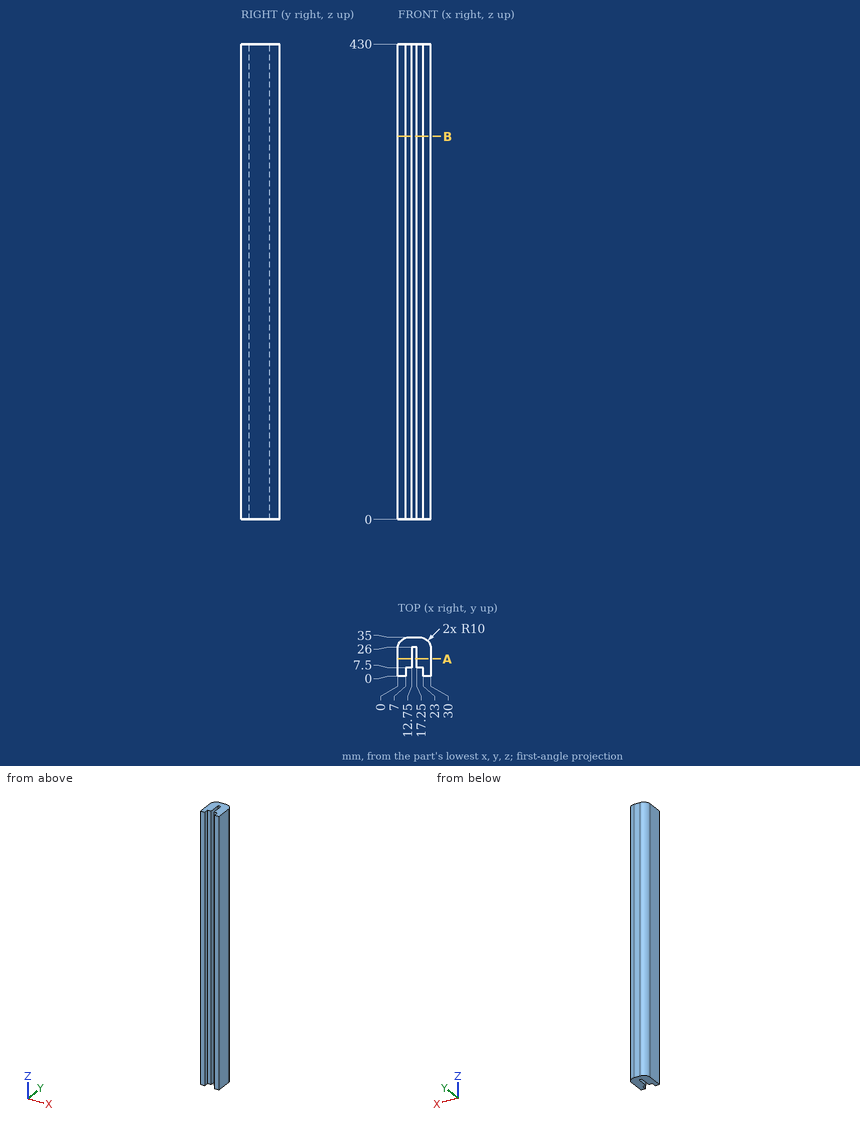
Part print with two shaded views. Sizes in mm from the minimum x, y, z corner. Give positions to 0.01 mm unless a question says otherwise; leave off trailing zeros. Order: outer loops, then holes, each group sorted by start corner. A loop starts at its lowest first (then second) coordinate and runs counter-clockwise, first axis right, second up. Notation, with made-up numbers: M 11,1.25 L 15,1.25 A5 cw 15,8.25 Z; hole C 21.25,27 d9. An arc over 180 degrees is marked long. Use one line per item in the form item = value.
1) Drop flat-ended pins along their axis: pin 1 (1.7 mm diameter, centred on x = 8.5, z = 141, fed in from -Y); pin 2 (1.5 mm diameter, centred on x = 9.5, y = 6.5, fed in from +Z). Give the stop position or say it passes through.
Calculated:
pin_1 = 7.5
pin_2 = through
2) Saw through at B-B (z = 346.5). Give the cut face in (x, y).
Calculated:
outline = M 0,0 L 7,0 L 7,7.5 L 12.75,7.5 L 12.75,26 L 17.25,26 L 17.25,7.5 L 23,7.5 L 23,0 L 30,0 L 30,25 A10 ccw 20,35 L 10,35 A10 ccw 0,25 Z
3) Probe probe 1 along X at (y, z) = (2.5, 143.5); probe 2 along X at (y, z) = (15.5, 348); probe 3 along Y at (x, z) = (15, 318.5). List the from-to ranges inside material, lowest first.
Calculated:
probe_1 = 0 to 7, 23 to 30
probe_2 = 0 to 12.75, 17.25 to 30
probe_3 = 26 to 35
4) Saw through at A-A (y = 15.5). Give the cut face in (x, z), plus the area to 3 significant figures.
Calculated:
outline = M 0,0 L 12.75,0 L 12.75,430 L 0,430 Z; M 17.25,0 L 30,0 L 30,430 L 17.25,430 Z
area = 11,000 mm2
